The figure shows three views and two pictorial views of one solid part (mm, origin at its lowest corner). Answer the questions. A direction names the side the tool comes from. Give positions to 0.01 mm unless a question says otherwise; leave off trailing zeros. Write each loop counter-clockwise with the first axis right and the second up, starting at its lowest first coordinate (ties: lowest second). Pieces come first, ordered by that corner, then holes. Notation, with made-up numbers: (3, -29.5) -> (30, -29.5) arc R23 cw to (30, -5.5) -> close; hole circle Ø9 at (63, -9). An arc over 180 degrees is marked (long way). Use a Markdown table: item, result.
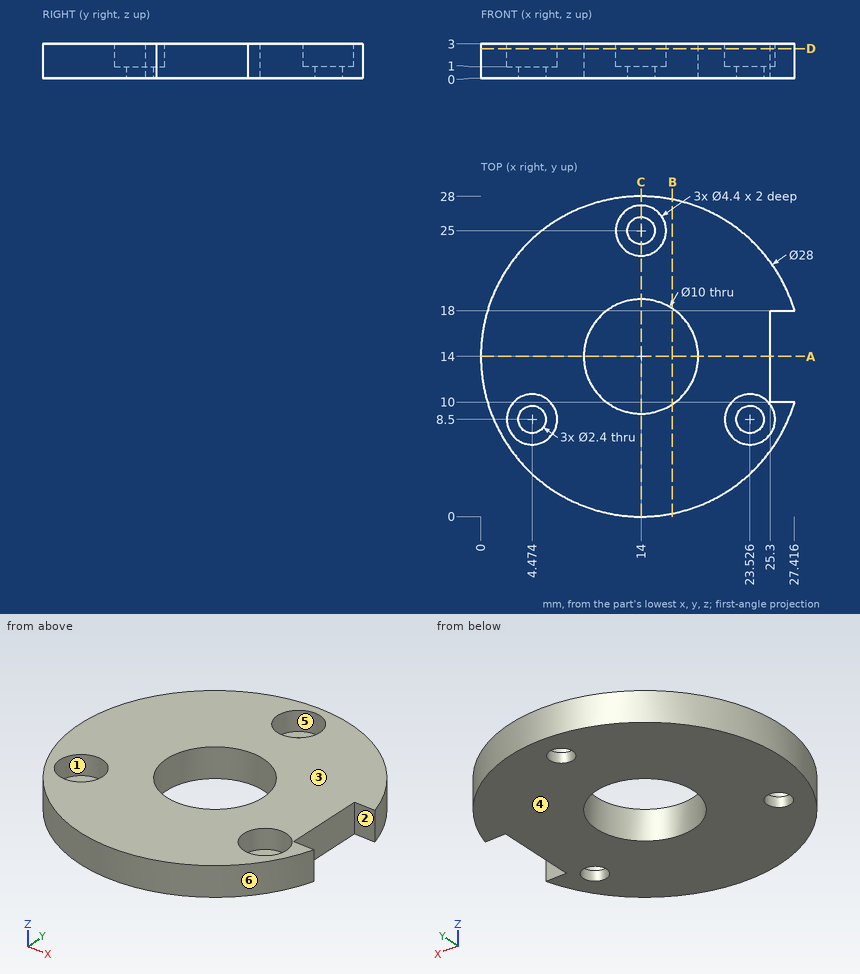
Item 1: Each of these flat-tipped pins is pushed along its axis until it touches: P1, Ø2, axis at x = 23, y = 7.5, coming from the +Z side; P2, Ø1, axis at x = 20.5, z = 0.5, coming from the +Y side; P3, Ø2, axis at x = 13, y = 16.5, coming from the +Z side; P4, Ø1.1, axis at x = 26, z = 2, coming from the -Y side (1 decimal). Where does it stop, or does it pass through?
Return value:
| item | result |
|---|---|
| P1 | z = 1 |
| P2 | y = 26.65 |
| P3 | through |
| P4 | y = 5.9 |
Item 2: A cutting plane is placed at D-D (z = 2.6). Give the vertices of the cut face in (x, y) (1 decimal).
Return value:
| item | result |
|---|---|
| outline | (25.3, 10) -> (25.3, 18) -> (27.4, 18) arc R14 ccw (long way) to (27.4, 10) -> close; hole circle Ø4.4 at (4.5, 8.5); hole circle Ø10 at (14, 14); hole circle Ø4.4 at (14, 25); hole circle Ø4.4 at (23.5, 8.5) |
Item 3: For a pull along Y with two mould halves and no side action, classify the marked faces 4, 5 and 6 as +Y half, -Y half, draft (parallel to the pull), parting line (faces both ways), or undercut.
Return value:
| item | result |
|---|---|
| face 4 | draft |
| face 5 | undercut |
| face 6 | parting line |
Item 4: A tool of negligible diameter and unlimited length cuts with its end or side. For the marked faces 1, 2 and 3, from which of +Z, -Z, +X, -X, +Y, -Y can it reach the whole face along a straight path? Write none if from no direction.
Return value:
| item | result |
|---|---|
| face 1 | +Z |
| face 2 | +Z, -Z, +X |
| face 3 | +Z, +X, -X, +Y, -Y |
Item 5: A cutting plane is placed at A-A (y = 14). Give the vertices of the cut face in (x, z).
Return value:
| item | result |
|---|---|
| outline | (0, 0) -> (9, 0) -> (9, 3) -> (0, 3) -> close; (19, 0) -> (25.3, 0) -> (25.3, 3) -> (19, 3) -> close |
Item 6: A cutting plane is placed at C-C (x = 14). Give the vertices of the cut face in (y, z).
Return value:
| item | result |
|---|---|
| outline | (0, 0) -> (9, 0) -> (9, 3) -> (0, 3) -> close; (19, 0) -> (23.8, 0) -> (23.8, 1) -> (22.8, 1) -> (22.8, 3) -> (19, 3) -> close; (26.2, 0) -> (28, 0) -> (28, 3) -> (27.2, 3) -> (27.2, 1) -> (26.2, 1) -> close |
Item 7: Straight lines are drawn through the part: line 1 along Y through (x, z) = (14, 0.5); line 2 along Y through (x, z) = (14, 1.5); line 3 along X through (y, z) = (6.75, 1.5) (1 decimal). For each, find the intervals that lie inside material, in ascending order. Write a range as [from, to].
Return value:
| item | result |
|---|---|
| line 1 | [0, 9], [19, 23.8], [26.2, 28] |
| line 2 | [0, 9], [19, 22.8], [27.2, 28] |
| line 3 | [2, 3.1], [5.8, 22.2], [24.9, 26] |
Item 8: A cutting plane is placed at B-B (x = 16.75). Give the vertices of the cut face in (y, z) (1 decimal).
Return value:
| item | result |
|---|---|
| outline | (0.3, 0) -> (9.8, 0) -> (9.8, 3) -> (0.3, 3) -> close; (18.2, 0) -> (27.7, 0) -> (27.7, 3) -> (18.2, 3) -> close |
